Can you work these out from the drawing? Everything is in mm from the part's minimum corner. Give positions to 0.01 mm unless a question says otherwise; leave off trailing zeros. Write each loop counter-clockwise with the first axis right and the second up, starting at its lowest first coordinate (ties: lowest second). Pieces come first, ordered by that corner, then holes. Notation, with made-up numbers: (78.25, 34) -> (135.25, 34) arc R21 ccw to (135.25, 46) -> close; hole circle Ø5 at (46.5, -3.75). An arc over 180 degrees is marked (long way). Answer as CSV lines item,"result". Start each with the question number.
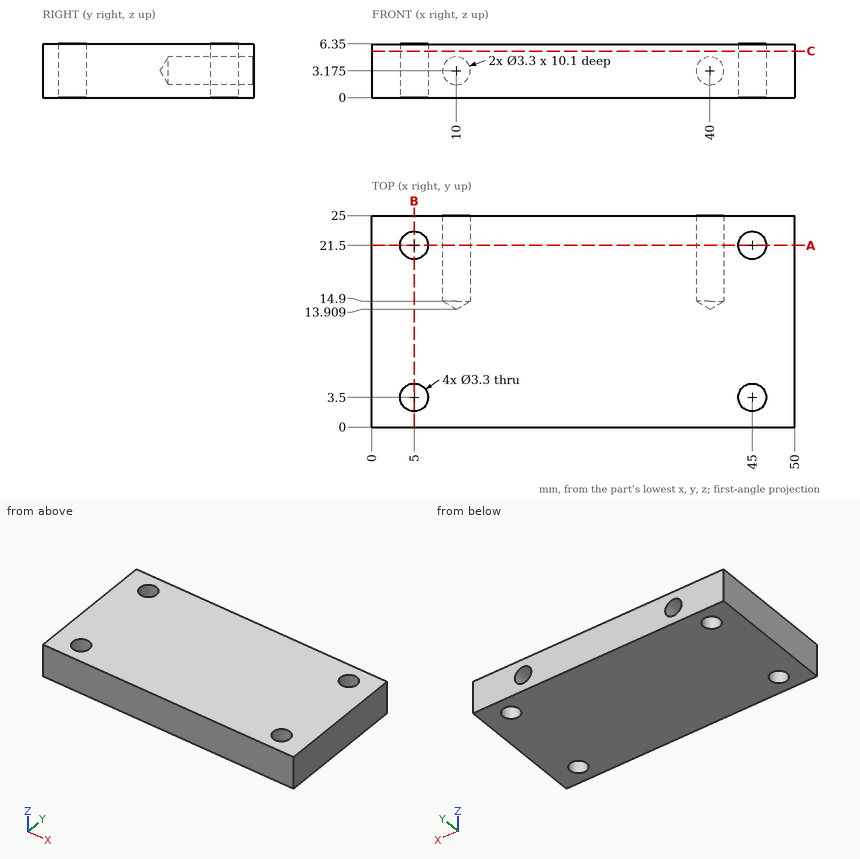
Item 1: If we section it at C-C (z = 5.5): Please give me the cut outline in (x, y), and give its area (3 significant figures).
Item 2: If we section it at A-A (y = 21.5): State how many separate pieces and enclosed holes the cut face has.
Item 3: If I drill on line 1 (Y direction, x = 5, z = 2); line 2 (X direction, y = 20.25, z = 1) (1 decimal); line 3 (X direction, y = 23, z = 1) (1 decimal), over which ranges is the centre line in solid material (lowest first)? Write a range as [from, to].
Item 4: I'm going to push a flat-ended pin straight in: pin 1 (3 mm diameter, centred on x = 40, z = 3.175, fed in from +Y). Where does the tip first touch, or does it pass through?
Item 5: If we section it at B-B (x = 5): Please give me the cut outline in (y, z), and give its area (3 significant figures).
Final values:
1,outline,"(0, 0) -> (50, 0) -> (50, 25) -> (0, 25) -> close; hole circle Ø3.3 at (5, 3.5); hole circle Ø3.3 at (5, 21.5); hole circle Ø3.3 at (45, 3.5); hole circle Ø3.3 at (45, 21.5)"
1,area,"1,220 mm2"
2,separate pieces,"3"
2,enclosed holes,"2"
3,line 1,"[0, 1.85], [5.15, 19.85], [23.15, 25]"
3,line 2,"[0, 3.9], [6.1, 43.9], [46.1, 50]"
3,line 3,"[0, 4.3], [5.7, 44.3], [45.7, 50]"
4,pin 1,"y = 14.81"
5,outline,"(0, 0) -> (1.85, 0) -> (1.85, 6.35) -> (0, 6.35) -> close; (5.15, 0) -> (19.85, 0) -> (19.85, 6.35) -> (5.15, 6.35) -> close; (23.15, 0) -> (25, 0) -> (25, 6.35) -> (23.15, 6.35) -> close"
5,area,"117 mm2"
